Input: dimensioned drawing with shaded views. Units: mm. Origin: part minimum x, y, z. A direction names the side the tool comes from. Give positions to 0.01 mm unless a question says otherwise; leave off trailing zeros. Write each loop counter-clockwise with the first axis right and the second up, starting at its lowest first coordinate (ties: lowest second). Pieces come first, ordered by that corner, then holes.
Q1. Section C-C (z = 10.5). Return the cut outline in (x, y).
Q2. Pin query (flat end, axial travel): pin 1 Ø12 at (y, z) = (19, 12.5) entering from -X; pin 2 Ø6 at (x, z) = (48, 4.5) entering from +Y; pin 3 Ø3 at (y, z) = (16, 6) entering from -X; pin 4 Ø10 at (x, y) = (29.5, 24.5) entering from +Z. Return the tip coordinate at first contact, or that it passes through.
Q3. Reachability of the marked faces 4 and 5 from +Z, -Z, +X, -X, +Y, -Y: full face, straight path, thin tool, end or side. Return the list, or none.
Q4. Section B-B (z = 6). Return the cut outline in (x, y), plus the area to 3 significant figures.
Q5. Section A-A (x = 31.75). Return the cut outline in (y, z).
Q6. Line query: line 1 (Y direction, x = 33.5, z = 24.5) (1 decimal); line 2 (Y direction, x = 38.5, z = 30); line 3 (X direction, y = 34.5, z = 18.5). Output: solid intervals per line, ascending.
Q7. Mould query, pull axis X, two halves, no side actions, for the marked faces 1, 2 and 3. Classes: +X half, -X half, draft (parallel to the pull), parting line (faces both ways), or undercut.
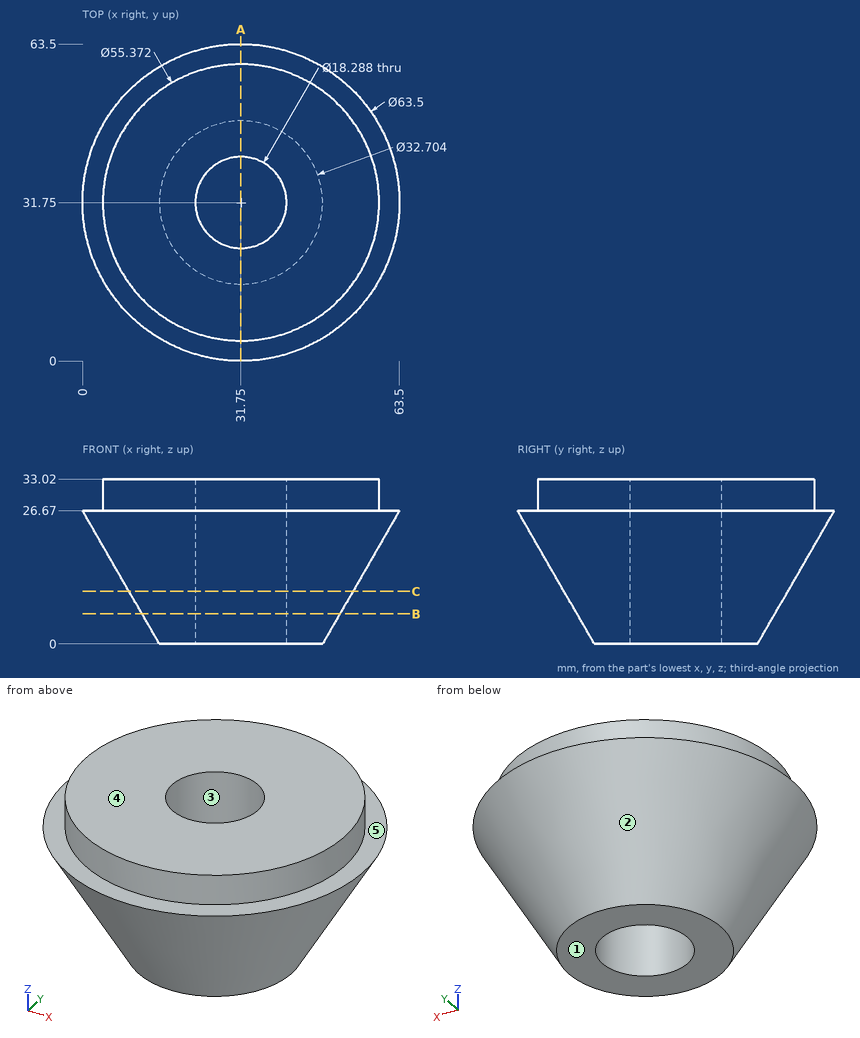
Computed:
1. outline: circle Ø44.83 at (31.75, 31.75); hole circle Ø18.29 at (31.75, 31.75)
2. pin 1: stops at x = 7.03
2. pin 2: stops at y = 46.17
2. pin 3: stops at x = 17.54
2. pin 4: stops at z = 33.02
3. face 4: +Z, +X, -X, +Y, -Y
3. face 5: +Z
4. outline: circle Ø39.63 at (31.75, 31.75); hole circle Ø18.29 at (31.75, 31.75)
4. area: 971 mm2
5. outline: (0, 26.67) - (15.4, 0) - (22.61, 0) - (22.61, 33.02) - (4.06, 33.02) - (4.06, 26.67) - close; (40.89, 0) - (48.1, 0) - (63.5, 26.67) - (59.44, 26.67) - (59.44, 33.02) - (40.89, 33.02) - close
6. line 1: y = 1.3 to 22.8, 40.7 to 62.2
6. line 2: y = 4.9 to 25.58, 37.92 to 58.6
6. line 3: x = 4.86 to 23.03, 40.47 to 58.64
7. face 1: draft
7. face 2: parting line
7. face 3: undercut
